The figure shows three views and two pictorial views of one solid part (mm, origin at its lowest corner). Answer the questions. A direction names the side the tool comes from. Give positions to 0.01 mm unless a question says otherwise; leave off trailing zeros. Write each loop counter-clockwise with the first axis right and the second up, starting at its lowest first coordinate (ties: lowest second). Pieces come first, ordered by that corner, then holes. Notation, with made-up numbers: (-10, 23) -> (-5, 23) arc R13 ccw to (-5, 38) -> close; hole circle Ø5 at (23.5, -1.5). An arc over 180 degrees is marked (long way). Use a Markdown table: item, result.
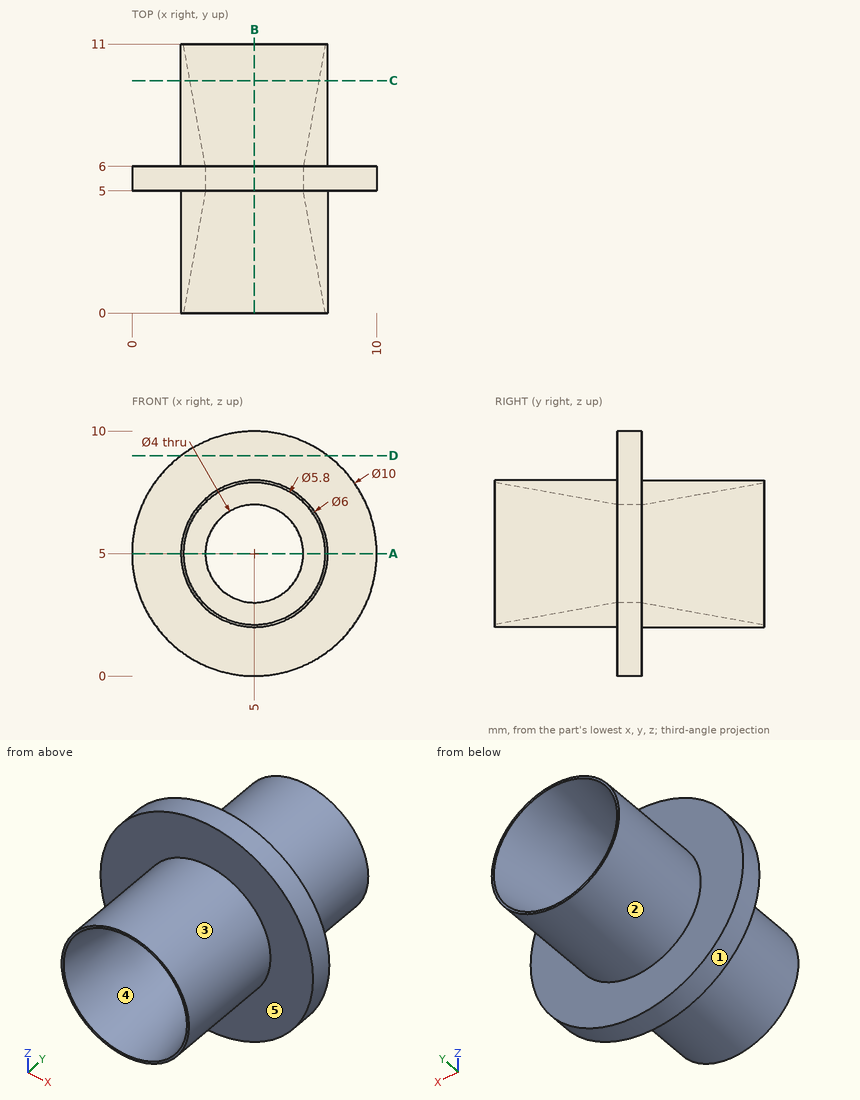
Item 1: A cutting plane is placed at A-A (z = 5). Give the vertices of the cut face in (x, y), then the cut area to 3 significant figures.
Return value:
| item | result |
|---|---|
| outline | (0, 5) -> (2, 5) -> (2, 0) -> (2.1, 0) -> (3, 5) -> (3, 6) -> (2.1, 11) -> (2, 11) -> (2, 6) -> (0, 6) -> close; (7, 5) -> (7.9, 0) -> (8, 0) -> (8, 5) -> (10, 5) -> (10, 6) -> (8, 6) -> (8, 11) -> (7.9, 11) -> (7, 6) -> close |
| area | 17.0 mm^2 |
Item 2: A cutting plane is placed at D-D (z = 9). Give the vertices of the cut face in (x, y), then the cut area to 3 significant figures.
Return value:
| item | result |
|---|---|
| outline | (2, 5) -> (8, 5) -> (8, 6) -> (2, 6) -> close |
| area | 6.00 mm^2 |
Item 3: A tool of negligible diameter and unlimited length cuts with its end or side. For the marked faces 1 and 2, from which of +Z, -Z, +X, -X, +Y, -Y can it reach the whole face along a straight path? Write none if from no direction.
Return value:
| item | result |
|---|---|
| face 1 | +Y, -Y |
| face 2 | +Y |
Item 4: Each of these flat-tipped pins is pushed along its axis until it touches: P1, Ø1.5, axis at x = 4.5, y = 1, coming from the -Z side; P2, Ø3, axis at y = 1.5, z = 7.5, coming from the +X side; P3, Ø4, axis at y = 9, z = 5.5, coming from the +X side. Where does it stop, or does it pass through?
Return value:
| item | result |
|---|---|
| P1 | z = 2 |
| P2 | x = 7.83 |
| P3 | x = 8 |
Item 5: A cutting plane is placed at C-C (y = 9.5). Give the vertices of the cut face in (x, z).
Return value:
| item | result |
|---|---|
| outline | circle Ø6 at (5, 5); hole circle Ø5.26 at (5, 5) |
Item 6: A cutting plane is placed at B-B (x = 5). Give the vertices of the cut face in (y, z).
Return value:
| item | result |
|---|---|
| outline | (0, 2) -> (5, 2) -> (5, 0) -> (6, 0) -> (6, 2) -> (11, 2) -> (11, 2.1) -> (6, 3) -> (5, 3) -> (0, 2.1) -> close; (0, 7.9) -> (5, 7) -> (6, 7) -> (11, 7.9) -> (11, 8) -> (6, 8) -> (6, 10) -> (5, 10) -> (5, 8) -> (0, 8) -> close |
Item 7: Straight lines are drawn through the part: line 1 along Z through (x, y) = (5, 5.85); line 2 along Y through (x, z) = (0.75, 3.25); line 3 along Z through (x, y) = (4.5, 7.25). For each, find the intervals that lie inside material, in ascending order. Write a range as [from, to].
Return value:
| item | result |
|---|---|
| line 1 | [0, 3], [7, 10] |
| line 2 | [5, 6] |
| line 3 | [2.04, 2.83], [7.17, 7.96] |
Item 8: For a pull along Z with two mould halves and no side action, classify the marked faces 3, 4 and 5 as +Z half, -Z half, draft (parallel to the pull), parting line (faces both ways), or undercut.
Return value:
| item | result |
|---|---|
| face 3 | parting line |
| face 4 | undercut |
| face 5 | draft |
